Read the model definition and answer for the solid it produces. Units are mm, in the model's axes. Face numbers are marked on the shaded views. Coordinates: 2 decimals unless noted, no trailing zeros. Write each loop counter-clockwise with the first axis right and the second up, starting at its lowest first coordinate (ties: lowest second). Pieces come first, ordered by that corner, then holes. Notation, with made-up numbers: (70, -34.5) -> (84, -34.5) arc R30 cw to (84, -11.5) -> close; hole circle Ø9 at (40.5, -2). An arc over 180 degrees is marked (long way). One line per item, written item: value. Start each with the question number.
1. Find section A-A, the plane y = -1.75. Write down the section's boundary in (x, z), and give its area (3 significant figures).
2. Consider line 1 along Y through (x, z) = (0, 16.5); line 2 along Y through (x, z) = (6, 10.25). Determine where each line is inside the solid, lowest interval first.
3. For a pull along Z with two mould halves and no side action, classify the marked faces 1, 2 and 3 as pulls with the +Z half, pulls with the -Z half, needs draft (parallel to the pull), parting line crosses it, or undercut.
4. Find section B-B, the plane x = -0.5. Write down the section's boundary in (y, z), and give its area (3 significant figures).
5. Find section C-C, the plane z = 5. Write down the section's boundary in (x, y), and give its area (3 significant figures).
6. Find section D-D, the plane y = 5.5. Write down the section's boundary in (x, z).
7. Given P1, Ø4, axis at x = 4, y = -5, coming from the -Z side; P2, Ø1.5, axis at x = 1.5, z = 4, coming from the -Y side; P3, Ø0.8, axis at x = 8.5, z = 0.5, coming from the -Y side; P4, Ø12, axis at x = 0, y = 0, coming from the -Z side, each flat-ended and moving along its own axis, determine where each tip first touches the part or whether it passes through.
```python
from build123d import *

# Parameters (mm, degrees)
F0_R     = 10
F0_R_2   = 7.5
F1_DEPTH = 25
F3_DEPTH = 25


with BuildPart() as f1:
    # F0 (on Top) → F1 (new body)
    with BuildSketch(Plane.XY):
        Circle(F0_R)
        Circle(F0_R_2, mode=Mode.SUBTRACT)
    extrude(amount=F1_DEPTH)

    # F2 (on Front) → F3 (cut)
    with BuildSketch(Plane.XZ):
        Polygon((0, 3.849256), (-10, 0), (0, 0), align=None)
        Polygon((0, 3.849256), (0, 0), (10, 0), align=None)
        Polygon((-10, 8.024929), (-10, 2.282619), (0, 6.373282), (0, 8.024929), align=None)
        Polygon((0, 8.024929), (0, 6.373282), (10, 2.369654), (10, 8.024929), align=None)
    extrude(amount=F3_DEPTH, mode=Mode.SUBTRACT)


solid = f1.part
```
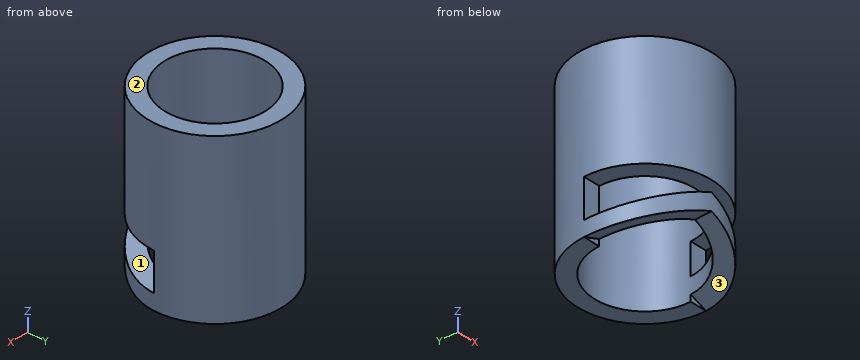
Answer block:
1. outline: (-9.85, 0.06) -> (-7.29, 1.04) -> (-7.29, 3.39) -> (-9.85, 2.35) -> close; (-9.85, 8.02) -> (-7.29, 8.02) -> (-7.29, 25) -> (-9.85, 25) -> close; (7.29, 1.04) -> (9.85, 0.06) -> (9.85, 2.43) -> (7.29, 3.45) -> close; (7.29, 8.02) -> (9.85, 8.02) -> (9.85, 25) -> (7.29, 25) -> close
1. area: 98.7 mm2
2. line 1: y = -10 to -7.5, 7.5 to 10
2. line 2: y = -8 to -4.5, 4.5 to 8
3. face 1: undercut
3. face 2: pulls with the +Z half
3. face 3: pulls with the -Z half
4. outline: (-9.99, 3.66) -> (-7.48, 3.66) -> (-7.48, 6.17) -> (-9.99, 6.17) -> close; (-9.99, 8.02) -> (-7.48, 8.02) -> (-7.48, 25) -> (-9.99, 25) -> close; (7.48, 0) -> (9.99, 0) -> (9.99, 25) -> (7.48, 25) -> close
4. area: 111 mm2
5. outline: (-10, 0) -> (-7.5, 0) arc R7.5 cw to (7.5, 0) -> (10, 0) arc R10 ccw to start; (-3.36, -9.42) arc R10 ccw to (3.43, -9.39) -> (3.43, -6.67) arc R7.5 cw to (-3.36, -6.71) -> close
5. area: 86.2 mm2
6. outline: (-8.35, 0) -> (-5.1, 0) -> (-5.1, 25) -> (-8.35, 25) -> close; (5.1, 0) -> (8.35, 0) -> (8.35, 25) -> (5.1, 25) -> close
7. P1: stops at z = 1.54
7. P2: stops at y = -9.97
7. P3: stops at y = -5.78
7. P4: passes through
